from build123d import *

# Parameters (mm, degrees)
F1_DEPTH    = 25.4
F2_R        = 12.7
F3_R        = 12.69999
F4_R        = 12.7
F5_T1_DEPTH = 76.2
F6_W        = 12.7
F6_H        = 17.3485226281
F7_DEPTH    = 25.4
F9_T1_DEPTH = 12.7
F10_R       = 5.08
F11_R       = 6.35
F12_DEPTH   = 12.7


# Not quite as in the source:
# - a fillet or chamfer that OpenCascade refuses, or shapes differently, is made with other operations: its cross-section is extruded or revolved along the edge and cut away or added
# - a fillet or chamfer is up to 0.001 mm smaller than in the source, because OpenCascade refuses the exact size
# - a feature of the source that left no trace in its solid (it failed there, or was rolled back) is left out


with BuildPart() as f1:
    # F0 (on Front) → F1 (new body)
    with BuildSketch(Plane.XZ):
        Polygon((0, 44.45), (0, 0), (57.15, 0), (57.15, 12.7), (12.7, 12.7), (12.7, 44.45), align=None)
    extrude(amount=F1_DEPTH)

    # F2
    f2_edges = [f1.edges().sort_by_distance(p)[0] for p in [
        (57.15, -25.4, 6.35),
    ]]
    fillet(f2_edges, radius=F2_R)

    # F3 (radius 12.7 in the source; OpenCascade refuses exactly that, so slightly less here)
    f3_edges = [f1.edges().sort_by_distance(p)[0] for p in [
        (57.15, 0, 6.35),
    ]]
    fillet(f3_edges, radius=F3_R)

    # F4
    f4_edges = [f1.edges().sort_by_distance(p)[0] for p in [
        (6.35, -25.4, 44.45),
    ]]
    fillet(f4_edges, radius=F4_R)

    # F5: fillet of radius 12.7 on 1 edges, made by hand

    # F5_s2 → F5_t1 (cut)
    with BuildSketch(Plane.YZ.offset(-31.75)):
        with BuildLine():
            ThreePointArc((-12.7, 44.45), (-3.7197438789, 40.7302561211), (0, 31.75))
            Line((0, 31.75), (0, 44.45))
            Line((0, 44.45), (-12.7, 44.45))
        make_face()
    extrude(amount=F5_T1_DEPTH, mode=Mode.SUBTRACT)

    # F6 (on face) → F7 (cut)
    with BuildSketch(Plane.YZ.offset(12.7)):
        with BuildLine():
            ThreePointArc((-12.7, 44.45), (-15.9870018728, 44.0172579939), (-19.05, 42.7485226281))
            Line((-19.05, 42.7485226281), (-6.35, 42.7485226281))
            ThreePointArc((-6.35, 42.7485226281), (-9.4129981272, 44.0172579939), (-12.7, 44.45))
        make_face()
        with Locations((-12.7, 34.074261314)):
            Rectangle(F6_W, F6_H)
    extrude(amount=-F7_DEPTH, mode=Mode.SUBTRACT)

    # F9: fillet of radius 12.7 on 2 edges, made by hand

    # F9_s2 → F9_t1 (join)
    with BuildSketch(Plane.YZ):
        with BuildLine():
            ThreePointArc((-19.05, 38.1), (-15.3302561211, 29.1197438789), (-6.35, 25.4))
            Line((-6.35, 25.4), (-19.05, 25.4))
            Line((-19.05, 25.4), (-19.05, 38.1))
        make_face()
        with BuildLine():
            ThreePointArc((-19.05, 25.4), (-10.0697438789, 29.1197438789), (-6.35, 38.1))
            Line((-6.35, 38.1), (-6.35, 25.4))
            Line((-6.35, 25.4), (-19.05, 25.4))
        make_face()
    extrude(amount=F9_T1_DEPTH)

    # F10
    f10_edges = [f1.edges().sort_by_distance(p)[0] for p in [
        (6.35, -12.7, 27.101477),
    ]]
    fillet(f10_edges, radius=F10_R)

    # F11 (on face) → F12 (cut)
    with BuildSketch(Plane.XY.offset(12.7)):
        with Locations((25.4, -12.7)):
            Circle(F11_R)
        with Locations((44.45, -12.7)):
            Circle(F11_R)
    extrude(amount=-F12_DEPTH, mode=Mode.SUBTRACT)


solid = f1.part
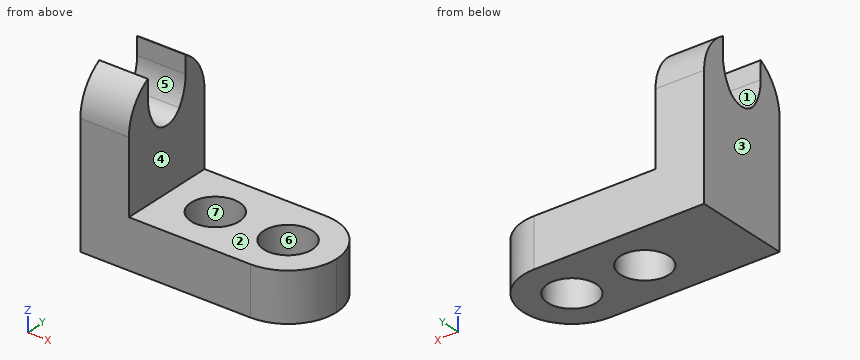
Part model, mm, in its own coordinate system. Face numbers are marked on the shaded views. A direction names the side the tool comes from. Coordinates: 2 decimals unless noted, no trailing zeros. Loops run counter-clockwise (first coordinate to the right, second up) from the corner with the lowest first, then second, coordinate; pieces in that order, holes last. Notation, with made-up numbers: (-23, -38.75) - (-18, -38.75) arc R25 cw to (-18, -6.75) - close; hole circle Ø6 at (63.25, 59.5). An arc over 180 degrees is marked (long way). Write each question's results on one line, items separated by ' | '. Start each with the question number.
Q1. Slice it at B-B on z = 10.5. Give the number of separate pieces and of enclosed holes in the cut face, and give its area (3 significant figures).
Q2. Slice it at D-D on x = 40.5. Give the cut face in (y, z).
Q3. Drop flat-ended pins along their axis: pin 1 Ø5 at (x, z) = (6, 41) entering from +Y; pin 2 Ø12.5 at (y, z) = (-9.5, 31.5) entering from +X; pin 3 Ø5 at (x, z) = (8.5, 40) entering from -Y; pin 4 Ø7.5 at (x, y) = (25.4, -12.7) entering from -Z. Give the stop position or say it passes through.
Q4. Which spindle directions (+Z, -Z, +X, -X, +Y, -Y) get a long thin tool onto all of the face, cutting with end or side? Do the marked faces 1, 2 and 3. Say none if no direction does.
Q5. Slice it at A-A on x = 25.4. Give the cut face in (y, z), and give its area (3 significant figures).
Q6. Probe line 1 along Y through (x, z) = (25.4, 8.25); line 2 along Z through (x, y) = (51, -6). List the from-to ranges inside material, lowest first.
Q7. Slice it at C-C on y = -18. Give the cut face in (x, z).
Q8. Two-plate mould, pull along X, no slides. Class the marked faces 4, 5, 6 and 7: +X half, -X half, draft (parallel to the pull), parting line (faces both ways), or undercut.
Answer:
1) separate pieces: 1 | enclosed holes: 2 | area: 1,130 mm2
2) outline: (-25.4, 0) - (-17.67, 0) - (-17.67, 12.7) - (-25.4, 12.7) - close; (-7.73, 0) - (0, 0) - (0, 12.7) - (-7.73, 12.7) - close
3) pin 1: stops at y = -1.94 | pin 2: stops at x = 12.7 | pin 3: stops at y = -24.02 | pin 4: passes through
4) face 1: +Z, +X, -X | face 2: +Z, +X, +Y, -Y | face 3: +Z, -Z, -X, +Y, -Y
5) outline: (-25.4, 0) - (-19.05, 0) - (-19.05, 12.7) - (-25.4, 12.7) - close; (-6.35, 0) - (0, 0) - (0, 12.7) - (-6.35, 12.7) - close | area: 161 mm2
6) line 1: y = -25.4 to -19.05, -6.35 to 0 | line 2: z = 0 to 12.7
7) outline: (0, 0) - (21.9, 0) - (21.9, 12.7) - (12.7, 12.7) - (12.7, 33.04) - (0, 33.04) - close; (28.9, 0) - (40.95, 0) - (40.95, 12.7) - (28.9, 12.7) - close; (47.95, 0) - (55.99, 0) - (55.99, 12.7) - (47.95, 12.7) - close
8) face 4: +X half | face 5: draft | face 6: undercut | face 7: undercut
